```python
from build123d import *

# Parameters (mm, degrees)
BOSS_EXTRUDE1_DEPTH = 10


with BuildPart() as part:
    # Sketch1 → Boss-Extrude1 (new body)
    with BuildSketch(Plane.XY):
        Polygon((28.479998469, 5.585850997), (28.479998469, -14.414149003), (-35.379946586, -14.414149003), (-35.379946586, -12.65984759), align=None)
        Polygon((27.479998469, 4.260121013), (27.479998469, -13.414149003), (8.794915094, -13.414149003), (8.794915094, -1.078474237), align=None, mode=Mode.SUBTRACT)
        Polygon((7.794915094, -1.364188523), (7.794915094, -13.414149003), (-10.083352731, -13.414149003), (-10.083352731, -6.472265045), align=None, mode=Mode.SUBTRACT)
        Polygon((-11.083352731, -6.75797933), (-11.083352731, -13.414149003), (-34.379946586, -13.414149003), align=None, mode=Mode.SUBTRACT)
    extrude(amount=BOSS_EXTRUDE1_DEPTH)


solid = part.part
```
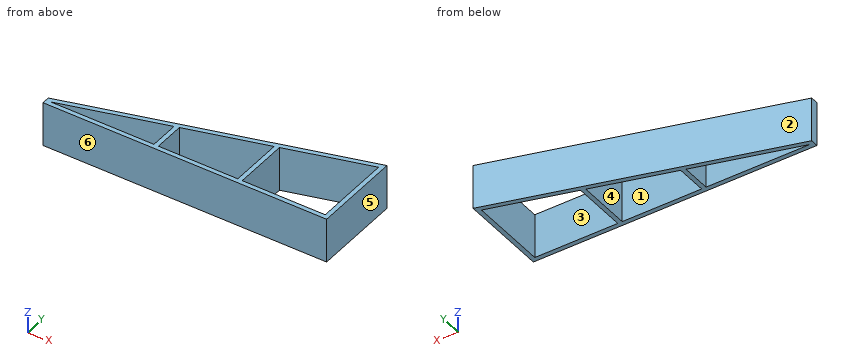
Check sheet for the modelled part. Datum: model origin and axes. Units: mm. Face numbers are marked on the shaded views. A direction names the side the tool comes from. Round coordinates to 2 decimals unless told otherwise and drop trailing zeros. Order: outer loops, then holes, each group sorted by start corner. A loop starts at its lowest first (then second) coordinate and runs counter-clockwise, first axis right, second up.
1) Section check C-C (x = -7.5). Record the boundary of the cut face in (y, z).
2) Mould release check, pull along X, two halves, no side actions. Record for the marked faces 3, 4, 5 and 6: +X half, -X half, draft (parallel to the pull), parting line (faces both ways), or undercut.
3) Section check B-B (y = -7.75). Record the boundary of the cut face in (x, z), and give its area (3 significant figures).
4) Go/stop test with flat-tipped pins: pin 1 Ø1.5 at (x, z) = (1, 4) entering from +Y; pin 2 Ø3 at (x, z) = (-23, 5) entering from +Y; pin 3 Ø5 at (x, z) = (-0.5, 5.5) entering from +Y. Record where each tip stops, or that it passes through.
5) Scan lines: line 1 (Y direction, x = 18, z = 4); line 2 (Y direction, x = 3.5, z = 7). Record each from-to range of solid material in increasing order.
6) Tool access check on the marked faces 1 and 2. Record the directions out of +Z, -Z, +X, -X, +Y, -Y that give a thin tool (end or side, any length) a straight path to the whole face; none if there is none.
7) Section check D-D (y = 3). Record the boundary of the cut face in (x, z), and give its area (3 significant figures).
8) Section check A-A (z = 4). Record the boundary of the cut face in (x, y).
Result:
1. outline: (-14.41, 0) - (-13.41, 0) - (-13.41, 10) - (-14.41, 10) - close; (-5.73, 0) - (-4.69, 0) - (-4.69, 10) - (-5.73, 10) - close
2. face 3: undercut
2. face 4: undercut
2. face 5: +X half
2. face 6: draft
3. outline: (-18.2, 0) - (-14.56, 0) - (-14.56, 10) - (-18.2, 10) - close; (-11.08, 0) - (-10.08, 0) - (-10.08, 10) - (-11.08, 10) - close; (7.79, 0) - (8.79, 0) - (8.79, 10) - (7.79, 10) - close; (27.48, 0) - (28.48, 0) - (28.48, 10) - (27.48, 10) - close
3. area: 66.4 mm2
4. pin 1: stops at y = -2.05
4. pin 2: stops at y = -8.69
4. pin 3: stops at y = -1.98
5. line 1: y = -14.41 to -13.41, 1.55 to 2.59
5. line 2: y = -14.41 to -13.41, -2.59 to -1.55
6. face 1: +Z, -Z
6. face 2: +Z, -Z, -X, +Y
7. outline: (19.43, 0) - (23.07, 0) - (23.07, 10) - (19.43, 10) - close; (27.48, 0) - (28.48, 0) - (28.48, 10) - (27.48, 10) - close
7. area: 46.4 mm2
8. outline: (-35.38, -14.41) - (28.48, -14.41) - (28.48, 5.59) - (-35.38, -12.66) - close; hole (-34.38, -13.41) - (-11.08, -13.41) - (-11.08, -6.76) - close; hole (-10.08, -13.41) - (7.79, -13.41) - (7.79, -1.36) - (-10.08, -6.47) - close; hole (8.79, -13.41) - (27.48, -13.41) - (27.48, 4.26) - (8.79, -1.08) - close
